```python
from build123d import *

# Parameters (mm, degrees)
SKETCH1_R           = 2.5
SKETCH1_R_2         = 1.250000001
SKETCH1_R_3         = 1.25
SKETCH1_R_4         = 2.1
SKETCH1_R_5         = 11
BOSS_EXTRUDE1_DEPTH = 2.5
CUT_EXTRUDE15_REACH = 140.384
SKETCH15_R          = 2.1
FILLET1_R           = 5
FILLET2_R           = 0.5
SKETCH21_R          = 2
SKETCH21_R_2        = 4
CUT_EXTRUDE21_DEPTH = 139.383525031
SKETCH22_W          = 40
SKETCH22_H          = 25
SKETCH22_R          = 4
BOSS_EXTRUDE2_DEPTH = 5
FILLET10_R          = 20
FILLET11_R          = 10


with BuildPart() as part:
    # Sketch1 → Boss-Extrude1 (new, symmetric)
    with BuildSketch(Plane.XY):
        with BuildLine():
            ThreePointArc((20.5, -64.4), (19.1, -63), (20.5, -61.6))
            Line((20.5, -61.6), (22.5, -61.6))
            ThreePointArc((22.5, -61.6), (23.9, -63), (22.5, -64.4))
            Line((22.5, -64.4), (22.5, -65))
            Line((22.5, -65), (30, -65))
            Line((30, -65), (30, 105))
            ThreePointArc((30, 105), (0, 135), (-30, 105))
            Line((-30, 105), (-30, -65))
            Line((-30, -65), (-22.5, -65))
            Line((-22.5, -65), (-22.5, -64.4))
            ThreePointArc((-22.5, -64.4), (-23.9, -63), (-22.5, -61.6))
            Line((-22.5, -61.6), (-20.5, -61.6))
            ThreePointArc((-20.5, -61.6), (-19.1, -63), (-20.5, -64.4))
            Line((-20.5, -64.4), (-20.5, -65))
            Line((-20.5, -65), (20.5, -65))
            Line((20.5, -65), (20.5, -64.4))
        make_face()
        with Locations((-21.5, -53)):
            Circle(SKETCH1_R, mode=Mode.SUBTRACT)
        with BuildLine():
            Line((-20.5, -48.4), (-22.5, -48.4))
            ThreePointArc((-22.5, -48.4), (-23.9, -47), (-22.5, -45.6))
            Line((-22.5, -45.6), (-20.5, -45.6))
            ThreePointArc((-20.5, -45.6), (-19.1, -47), (-20.5, -48.4))
        make_face(mode=Mode.SUBTRACT)
        with Locations((21.5, -53)):
            Circle(SKETCH1_R, mode=Mode.SUBTRACT)
        with BuildLine():
            ThreePointArc((22.5, -45.6), (23.9, -47), (22.5, -48.4))
            Line((22.5, -48.4), (20.5, -48.4))
            ThreePointArc((20.5, -48.4), (19.1, -47), (20.5, -45.6))
            Line((20.5, -45.6), (22.5, -45.6))
        make_face(mode=Mode.SUBTRACT)
        with Locations((-27.222941247, 58.222284236)):
            Circle(SKETCH1_R_2, mode=Mode.SUBTRACT)
        with Locations((-22.222941247, 58.222284236)):
            Circle(SKETCH1_R_2, mode=Mode.SUBTRACT)
        with Locations((-11.076110698, 74.544863638)):
            Circle(SKETCH1_R_3, mode=Mode.SUBTRACT)
        with Locations((-6.51035255, 76.582963865)):
            Circle(SKETCH1_R_3, mode=Mode.SUBTRACT)
        with Locations((-20, 105)):
            Circle(SKETCH1_R_4, mode=Mode.SUBTRACT)
        with Locations((0, 105)):
            Circle(SKETCH1_R_5, mode=Mode.SUBTRACT)
        with Locations((0, 125)):
            Circle(SKETCH1_R_4, mode=Mode.SUBTRACT)
        with Locations((0, 85)):
            Circle(SKETCH1_R_4, mode=Mode.SUBTRACT)
        with Locations((20, 105)):
            Circle(SKETCH1_R_4, mode=Mode.SUBTRACT)
    extrude(amount=BOSS_EXTRUDE1_DEPTH, both=True)

    # Sketch15 → Cut-Extrude15 (cut, up to next)
    with BuildSketch(Plane(origin=(0, 0, -2.5), x_dir=(-1, 0, 0), z_dir=(0, 0, -1)), mode=Mode.PRIVATE) as cut_extrude15_sk1:
        with Locations((20, -30)):
            Circle(SKETCH15_R)
    cut_extrude15_tool1 = extrude(cut_extrude15_sk1.sketch, amount=-CUT_EXTRUDE15_REACH, mode=Mode.PRIVATE) & part.part
    # Sketch15 → Cut-Extrude15 (cut, up to next)
    with BuildSketch(Plane(origin=(0, 0, -2.5), x_dir=(-1, 0, 0), z_dir=(0, 0, -1)), mode=Mode.PRIVATE) as cut_extrude15_sk2:
        with Locations((-15, -30)):
            Circle(SKETCH15_R)
    cut_extrude15_tool2 = extrude(cut_extrude15_sk2.sketch, amount=-CUT_EXTRUDE15_REACH, mode=Mode.PRIVATE) & part.part
    # Sketch15 → Cut-Extrude15 (cut, up to next)
    with BuildSketch(Plane(origin=(0, 0, -2.5), x_dir=(-1, 0, 0), z_dir=(0, 0, -1)), mode=Mode.PRIVATE) as cut_extrude15_sk3:
        with Locations((-20, 45)):
            Circle(SKETCH15_R)
    cut_extrude15_tool3 = extrude(cut_extrude15_sk3.sketch, amount=-CUT_EXTRUDE15_REACH, mode=Mode.PRIVATE) & part.part
    # Sketch15 → Cut-Extrude15 (cut, up to next)
    with BuildSketch(Plane(origin=(0, 0, -2.5), x_dir=(-1, 0, 0), z_dir=(0, 0, -1)), mode=Mode.PRIVATE) as cut_extrude15_sk4:
        with Locations((20, 45)):
            Circle(SKETCH15_R)
    cut_extrude15_tool4 = extrude(cut_extrude15_sk4.sketch, amount=-CUT_EXTRUDE15_REACH, mode=Mode.PRIVATE) & part.part
    add(cut_extrude15_tool1.solids().sort_by_distance((-20, -30, -2.5))[0], mode=Mode.SUBTRACT)
    add(cut_extrude15_tool2.solids().sort_by_distance((15, -30, -2.5))[0], mode=Mode.SUBTRACT)
    add(cut_extrude15_tool3.solids().sort_by_distance((20, 45, -2.5))[0], mode=Mode.SUBTRACT)
    add(cut_extrude15_tool4.solids().sort_by_distance((-20, 45, -2.5))[0], mode=Mode.SUBTRACT)

    # Fillet1
    fillet1_edges = [part.edges().sort_by_distance(p)[0] for p in [
        (-30, -65, 0),
        (30, -65, 0),
    ]]
    fillet(fillet1_edges, radius=FILLET1_R)

    # Fillet2
    # the kernel refuses this fillet: 0.5 mm, written as the material it takes off along each edge
    with BuildSketch(Plane(origin=(22.5, -65, -3.75), x_dir=(1, 0, 0), z_dir=(0, 0, 1)), Plane(origin=(-20.5, -65, 3.75), x_dir=(0, 1, 0), z_dir=(0, 0, -1))) as fillet2_piece_1:
        with BuildLine():
            CenterArc((FILLET2_R, FILLET2_R), FILLET2_R, 180, 90)
            Line((0, FILLET2_R), (0, 0))
            Line((0, 0), (FILLET2_R, 0))
        make_face()
    extrude(amount=7.5, mode=Mode.SUBTRACT)
    with BuildSketch(Plane(origin=(22.5, -64.4, -3.582575695), x_dir=(0, -1, 0), z_dir=(0, 0, 1))) as fillet2_piece_2:
        with BuildLine():
            CenterArc((0.433030278, 0.5), FILLET2_R, 195.25752329, 74.74247671)
            ThreePointArc((-0.049346111, 0.368421053), (-0.012391366, 0.185855529), (0, 0))
            Line((0, 0), (0.433030278, 0))
        make_face()
    extrude(amount=7.16515139, mode=Mode.SUBTRACT)
    with BuildSketch(Plane(origin=(20.5, -64.4, -3.582575695), x_dir=(0, -1, 0), z_dir=(0, 0, 1)), Plane(origin=(-22.5, -64.4, -3.582575695), x_dir=(0, -1, 0), z_dir=(0, 0, 1))) as fillet2_piece_3:
        with BuildLine():
            CenterArc((0.433030278, -0.5), FILLET2_R, 90, 74.74247671)
            ThreePointArc((-0.049346111, -0.368421053), (-0.012391366, -0.185855529), (0, 0))
            Line((0, 0), (0.433030278, 0))
        make_face()
    extrude(amount=7.16515139, mode=Mode.SUBTRACT)
    with BuildSketch(Plane(origin=(20.5, -65, -3.75), x_dir=(-1, 0, 0), z_dir=(0, 0, 1)), Plane(origin=(-22.5, -65, -3.75), x_dir=(-1, 0, 0), z_dir=(0, 0, 1))) as fillet2_piece_4:
        with BuildLine():
            CenterArc((FILLET2_R, -FILLET2_R), FILLET2_R, 90, 90)
            Line((0, -FILLET2_R), (0, 0))
            Line((0, 0), (FILLET2_R, 0))
        make_face()
    extrude(amount=7.5, mode=Mode.SUBTRACT)
    with BuildSketch(Plane(origin=(-20.5, -64.4, 3.582575695), x_dir=(0.9911490245884916, 0.1327539493095473, 0), z_dir=(0, 0, -1))) as fillet2_piece_5:
        with BuildLine():
            CenterArc((0.438088033, 0.495574512), FILLET2_R, 187.628761645, 74.74247671)
            Line((-0.05748648, 0.429197538), (0, 0))
            ThreePointArc((0, 0), (0.185855529, 0.012391366), (0.371711058, 0))
        make_face()
    extrude(amount=7.16515139, mode=Mode.SUBTRACT)

    # Sketch21 → Cut-Extrude21 (cut, through all)
    with BuildSketch(Plane.XY.offset(2.5)):
        with Locations((-20, -3.840572854)):
            Circle(SKETCH21_R)
        with Locations((-10, -3.840572854)):
            Circle(SKETCH21_R)
        with Locations((-15, 16.159427146)):
            Circle(SKETCH21_R)
        with Locations((20, 16.159427146)):
            Circle(SKETCH21_R_2)
    extrude(amount=-CUT_EXTRUDE21_DEPTH, mode=Mode.SUBTRACT)

    # Sketch22 → Boss-Extrude2 (add)
    with BuildSketch(Plane.XY.offset(2.5)):
        with Locations((50, 37.5)):
            Rectangle(SKETCH22_W, SKETCH22_H)
        with Locations((58, 35)):
            Circle(SKETCH22_R, mode=Mode.SUBTRACT)
    extrude(amount=-BOSS_EXTRUDE2_DEPTH)

    # Fillet10
    fillet10_edges = [part.edges().sort_by_distance(p)[0] for p in [
        (30, 25, 0),
        (30, 50, 0),
    ]]
    fillet(fillet10_edges, radius=FILLET10_R)

    # Fillet11
    fillet11_edges = [part.edges().sort_by_distance(p)[0] for p in [
        (70, 50, 0),
        (70, 25, 0),
    ]]
    fillet(fillet11_edges, radius=FILLET11_R)


solid = part.part
```
Design review of the part built by this model. Coordinates are the model's own, in mm. A direction names the side the tool comes from. Give positions to 0.01 mm unless a question says otherwise; leave off trailing zeros. Write each loop counter-clockwise with the first axis right and the second up, starting at its lowest first coordinate (ties: lowest second). Pieces come first, ordered by that corner, then holes.
(1) Add section C-C (y = 2.5). Give the boundary of the cut face in (x, z), and give its area (3 significant figures).
Checked values:
outline: (-30, -2.5) - (30, -2.5) - (30, 2.5) - (-30, 2.5) - close
area: 300 mm2
(2) Clearance check with flat-ended pins moving along their axes: pin 1 Ø1.5 at (x, z) = (48, 1) entering from -Y; pin 2 Ø2.5 at (x, z) = (53.5, 1) entering from -Y; pin 3 Ø2 at (x, y) = (-6.51, 76.58) entering from -Z; pin 4 Ø6.5 at (x, y) = (0, 125) entering from +Z. State where each tip first meets the part, or that it passes through.
Checked values:
pin 1: stops at y = 24.81
pin 2: stops at y = 25
pin 3: passes through
pin 4: stops at z = 2.5
(3) Add section D-D (z = 1.5). Give the number of separate pieces and of enclosed holes in the cut face, and give its area (3 significant figures).
Checked values:
separate pieces: 1
enclosed holes: 22
area: 12,000 mm2
(4) Mouldability with a two-part tool opening along Y and no side actions: class faces 1 (the face through (35.703, 56.014, -0.035)), 2 (the face through (-19.031, 103.137, -0.035)), 3 (the face through (30, -28, 0)) as +Y half, -Y half, draft (parallel to the pull), parting line (faces both ways), or undercut.
Checked values:
face 1: +Y half
face 2: undercut
face 3: draft
(5) Add section A-A (y = 125). Give the boundary of the cut face in (x, z), and give its area (3 significant figures).
Checked values:
outline: (-22.36, -2.5) - (-2.1, -2.5) - (-2.1, 2.5) - (-22.36, 2.5) - close; (2.1, -2.5) - (22.36, -2.5) - (22.36, 2.5) - (2.1, 2.5) - close
area: 203 mm2
(6) Add section B-B (x = -15). Give the boundary of the cut face in (y, z).
Checked values:
outline: (-65, -2.5) - (14.16, -2.5) - (14.16, 2.5) - (-65, 2.5) - close; (18.16, -2.5) - (130.98, -2.5) - (130.98, 2.5) - (18.16, 2.5) - close
(7) Tool access review of faces 4 (the face through (-1.666, 83.722, -0.035)), 5 (the face through (55, 50, 0)), 6 (the face through (55, 25, 0)): name each direction out of +Z, -Z, +X, -X, +Y, -Y from which nothing blocks a thin tool from reaching the whole face with its end or side.
Checked values:
face 4: +Z, -Z
face 5: +Z, -Z, +X, +Y
face 6: +Z, -Z, +X, -Y
(8) Wall thickness on line 1 along Y through (x, z) = (16.5, 0.2); line 2 along X through (y, z) = (106, 0.65); line 3 along Y through (x, z) = (61.5, -0.65): over which ranges is each line inside the solid? List them lowest first.
Checked values:
line 1: y = -65 to -31.47, -28.53 to 14.22, 18.1 to 130.05
line 2: x = -29.98 to -21.85, -18.15 to -10.95, 10.95 to 18.15, 21.85 to 29.98
line 3: y = 25.11 to 33.06, 36.94 to 49.89
